Part print with two shaded views. Sizes in mm from the minimum x, y, z corner. Round coordinates to 2 decimals unless told otherwise and drop trailing zeros. Write each loop counter-clockwise with the first axis right and the second up, starting at its lowest first coordinate (ties: lowest second). Pieces come first, ordered by that corner, then holes. Notation, with made-up numbers: (46, 46) -> (60, 46) arc R9 cw to (60, 54) -> close; hole circle Ø3 at (-28, -37.75). An arc over 180 degrees is marked (long way). Put each result on its own line as item: value. Start each with the question number.
1. Saw through at B-B on z = 6.5. List the corners of the cut face in (x, y).
2. Saw through at A-A on x = 21.31. List the corners of the cut face in (y, z).
3. Drill centre lines: line 1 (X direction, y = 3.5, z = 3.5); line 2 (X direction, y = 2.5, z = 5.25); line 3 (Y direction, x = 13.52, z = 7.35). Where is each one in solid material? Low to high. Write a range as from..to.
4. Saw through at C-C on y = 5. State how many separate pieces and enclosed holes the cut face has, and give its area (3 significant figures).
5. Saw through at D-D on x = 15.5. List the corners of the cut face in (y, z).
6. Pull direction Y, two halves, no side cores. Call the marked faces 1, 2, 3 and 4: pulls with the +Y half, pulls with the -Y half, needs draft (parallel to the pull), parting line crosses it, or undercut.
7. Flat gauge pins, fed straight in: P1, Ø3, axis at x = 12, y = 5, coming from the +Z side; P2, Ø3, axis at x = 20, y = 4, coming from the +Z side. Where does each tip first touch, or does it go through?
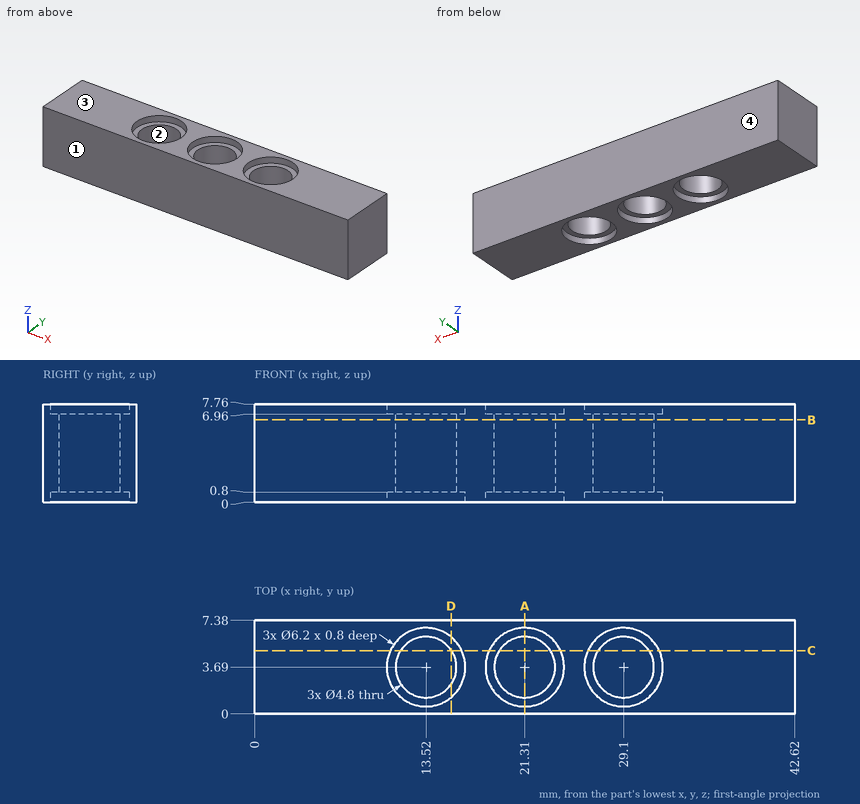
Return value:
1. outline: (0, 0) -> (42.62, 0) -> (42.62, 7.38) -> (0, 7.38) -> close; hole circle Ø4.8 at (13.52, 3.69); hole circle Ø4.8 at (21.31, 3.69); hole circle Ø4.8 at (29.1, 3.69)
2. outline: (0, 0) -> (0.59, 0) -> (0.59, 0.8) -> (1.29, 0.8) -> (1.29, 6.96) -> (0.59, 6.96) -> (0.59, 7.76) -> (0, 7.76) -> close; (6.09, 0.8) -> (6.79, 0.8) -> (6.79, 0) -> (7.38, 0) -> (7.38, 7.76) -> (6.79, 7.76) -> (6.79, 6.96) -> (6.09, 6.96) -> close
3. line 1: x = 0..11.13, 15.91..18.92, 23.7..26.71, 31.49..42.62
3. line 2: x = 0..11.44, 15.6..19.23, 23.39..27.02, 31.18..42.62
3. line 3: y = 0..0.59, 6.79..7.38
4. separate pieces: 4
4. enclosed holes: 0
4. area: 229 mm^2
5. outline: (0, 0) -> (1.3, 0) -> (1.3, 0.8) -> (2.33, 0.8) -> (2.33, 6.96) -> (1.3, 6.96) -> (1.3, 7.76) -> (0, 7.76) -> close; (5.05, 0.8) -> (6.08, 0.8) -> (6.08, 0) -> (7.38, 0) -> (7.38, 7.76) -> (6.08, 7.76) -> (6.08, 6.96) -> (5.05, 6.96) -> close
6. face 1: pulls with the -Y half
6. face 2: undercut
6. face 3: needs draft
6. face 4: pulls with the +Y half
7. P1: stops at z = 7.76
7. P2: stops at z = 6.96
